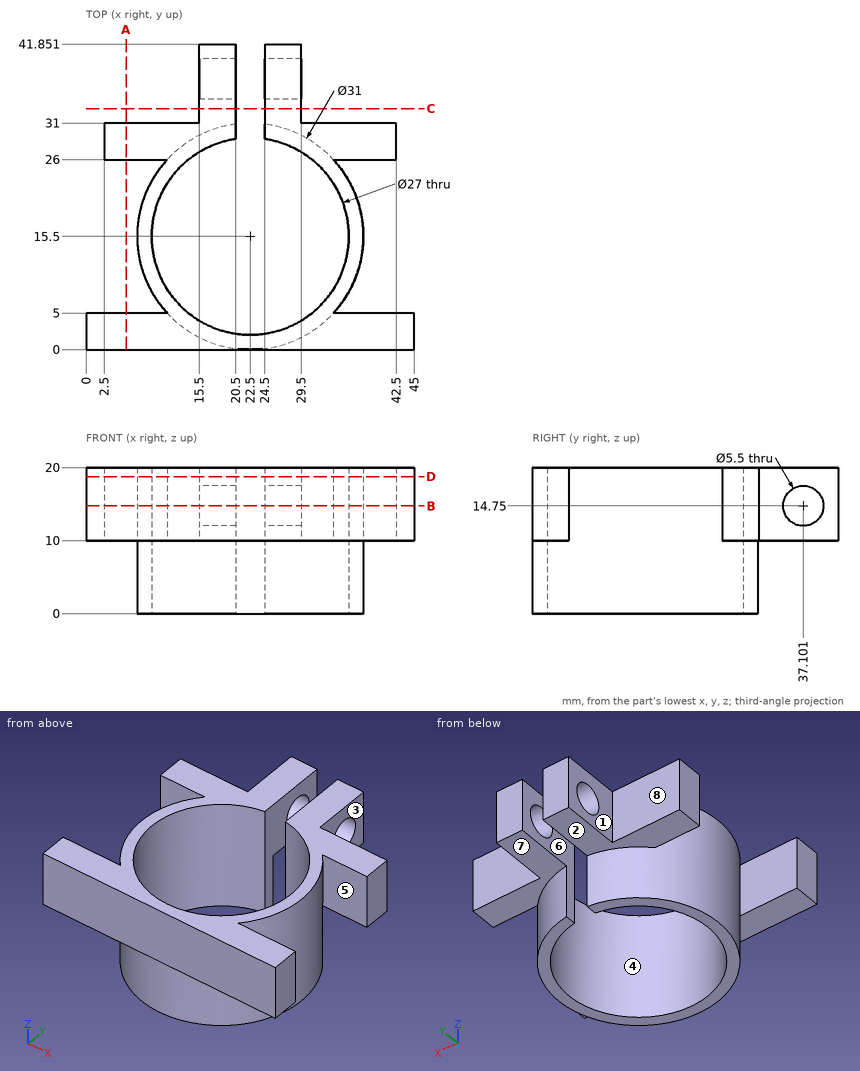
Drawing for the job (mm, zero at the part's lowest x, y, z). A direction names the side the tool comes from. Give positions to 0.01 mm unless a question says otherwise; leave off trailing zeros. Loops run counter-clockwise (first coordinate to the right, second up) from the corner with the lowest first, then second, coordinate; pieces in that order, holes last.
1) Two-plate mould, pull along X, no slides. Class the marked faces 1, 2, 3 and 4: released by +X, released by -X, zero draft, split by the parting line, or undercut.
Values follow:
face 1: released by -X
face 2: zero draft
face 3: released by +X
face 4: undercut
2) Band-saw the part on C-C on y = 33. List the corners of the cut face in (x, z), then the cut area to 3 significant figures.
Values follow:
outline: (15.5, 10) - (20.5, 10) - (20.5, 20) - (15.5, 20) - close; (24.5, 10) - (29.5, 10) - (29.5, 20) - (24.5, 20) - close
area: 100 mm2
3) Band-saw the part on B-B on z = 14.75. List the corners of the cut face in (x, y), then the cut area to 3 significant figures.
Values follow:
outline: (0, 0) - (45, 0) - (45, 5) - (33.9, 5) arc R15.5 ccw to (33.9, 26) - (42.5, 26) - (42.5, 31) - (29.5, 31) - (29.5, 34.35) - (24.5, 34.35) - (24.5, 28.85) arc R13.5 cw (long way) to (20.5, 28.85) - (20.5, 34.35) - (15.5, 34.35) - (15.5, 31) - (2.5, 31) - (2.5, 26) - (11.1, 26) arc R15.5 ccw to (11.1, 5) - (0, 5) - close; (15.5, 39.85) - (20.5, 39.85) - (20.5, 41.85) - (15.5, 41.85) - close; (24.5, 39.85) - (29.5, 39.85) - (29.5, 41.85) - (24.5, 41.85) - close
area: 495 mm2
4) Band-saw the part on D-D on z = 18.75. List the corners of the cut face in (x, y).
Values follow:
outline: (0, 0) - (45, 0) - (45, 5) - (33.9, 5) arc R15.5 ccw to (33.9, 26) - (42.5, 26) - (42.5, 31) - (29.5, 31) - (29.5, 41.85) - (24.5, 41.85) - (24.5, 28.85) arc R13.5 cw (long way) to (20.5, 28.85) - (20.5, 41.85) - (15.5, 41.85) - (15.5, 31) - (2.5, 31) - (2.5, 26) - (11.1, 26) arc R15.5 ccw to (11.1, 5) - (0, 5) - close
5) Band-saw the part on A-A on x = 5.5. List the corners of the cut face in (y, z).
Values follow:
outline: (0, 10) - (5, 10) - (5, 20) - (0, 20) - close; (26, 10) - (31, 10) - (31, 20) - (26, 20) - close
6) 3-axis set-ups, long thin cutter, end or side, ignore diameter. For the marked faces 5, 6, 7 and 8: which of +Z, -Z, +X, -X, +Y, -Y reach the whole face in a straight line?
Values follow:
face 5: +Z, -Z, +X
face 6: +Z, -Z, +Y
face 7: -Z, +X, +Y
face 8: +Z, -Z, -X, +Y
7) Probe line 1 along Z through (x, y) = (20, 34); line 2 along Y through (x, z) = (22.5, 11.5); line 3 along Y through (x, z) = (20, 16). List the from-to ranges inside material, lowest first.
Values follow:
line 1: z = 10 to 20
line 2: y = 0 to 2
line 3: y = 0 to 2.23, 28.77 to 34.65, 39.55 to 41.85
8) Drop flat-ended pins along their axis: P1, Ø1, axis at x = 31, z = 7.5, coming from the +Y side; P2, Ø3, axis at x = 37, z = 15.5, coming from the +Y side; P3, Ø5, axis at x = 34.5, y = 31, coming from the -Z side; P4, Ø4.5, axis at y = 37.1, z = 14.75, coming from the +X side. Give the stop position or say it passes through.
Values follow:
P1: stops at y = 28.78
P2: stops at y = 31
P3: stops at z = 10
P4: passes through
